Can you work these out from the model? Positions are in its coordinate system, mm. A direction names the side the tool comes from. Coordinates: 2 decimals unless noted, no trailing zeros. Loops run counter-clockwise (first coordinate to the right, second up) from the corner with the lowest first, then second, coordinate; pieces in that order, holes last.
```python
from build123d import *

# Parameters (mm, degrees)
SKETCH_1_R      = 23.5
EXTRUDE_1_DEPTH = 8
EXTRUDE_2_DEPTH = 70
FILLET_1_R      = 3
FILLET_2_R      = 3
EXTRUDE_3_DEPTH = 4


with BuildPart() as part:
    # 草图1 → 凸台-拉伸1 (new body)
    with BuildSketch(Plane.XY):
        with BuildLine():
            Line((30, -32.5), (-30, -32.5))
            Line((-30, -32.5), (-30, 0))
            ThreePointArc((-30, 0), (0, 30), (30, 0))
            Line((30, 0), (30, -32.5))
        make_face()
        Circle(SKETCH_1_R, mode=Mode.SUBTRACT)
    extrude(amount=EXTRUDE_1_DEPTH)

    # 草图2 → 凸台-拉伸2 (add)
    with BuildSketch(Plane(origin=(30, 0, 0), x_dir=(0, 0, -1), z_dir=(1, 0, 0))):
        Polygon((1, -32.5), (4, -32.5), (4, -27.5), (-12, -27.5), (-12, -32.5), (-9, -32.5), (-9, -42.5), (-19, -42.5), (-19, -47.5), (11, -47.5), (11, -42.5), (1, -42.5), align=None)
    extrude_2 = extrude(amount=-EXTRUDE_2_DEPTH)

    # 镜向1: 凸台-拉伸2 across plane
    add(extrude_2.mirror(Plane.ZY))

    # 圆角1
    fillet_1_edges = [part.edges().sort_by_distance(p)[0] for p in [
        (30, -13.75, 0),
        (30, -13.75, 8),
        (0, -27.5, 0),
        (-30, -27.5, 4),
        (0, -27.5, 8),
        (0, 30, 8),
        (-30, -13.75, 0),
        (0, 30, 0),
        (30, -27.5, 4),
        (-30, -13.75, 8),
    ]]
    fillet(fillet_1_edges, radius=FILLET_1_R)

    # 圆角2
    fillet_2_edges = [part.edges().sort_by_distance(p)[0] for p in [
        (-40, -47.5, 4),
        (0, -47.5, -11),
        (0, -47.5, 19),
        (40, -47.5, 4),
    ]]
    fillet(fillet_2_edges, radius=FILLET_2_R)

    # 草图4 → 凸台-拉伸3 (add, symmetric)
    with BuildSketch(Plane.XY.offset(4)):
        with BuildLine():
            Line((7.5, -47.5), (5, -47.5))
            Line((5, -47.5), (5, -52.5))
            ThreePointArc((5, -52.5), (0, -57.5), (-5, -52.5))
            Line((-5, -52.5), (-5, -47.5))
            Line((-5, -47.5), (-7.5, -47.5))
            Line((-7.5, -47.5), (-7.5, -52.5))
            ThreePointArc((-7.5, -52.5), (-6.18240924, -56.745917567), (-2.692582404, -59.5))
            Line((-2.692582404, -59.5), (2.692582404, -59.5))
            ThreePointArc((2.692582404, -59.5), (6.18240924, -56.745917567), (7.5, -52.5))
            Line((7.5, -52.5), (7.5, -47.5))
        make_face()
    extrude(amount=EXTRUDE_3_DEPTH, both=True)


solid = part.part
```
(1) I want a section at C-C on x = -35. Write out the boundary of the cut face in (y, z), then the cut area to 3 significant figures.
Check values:
outline: (-47.5, -8) arc R3 ccw to (-44.5, -11) - (-42.5, -11) - (-42.5, -1) - (-32.5, -1) - (-32.5, -4) - (-27.5, -4) - (-27.5, 12) - (-32.5, 12) - (-32.5, 9) - (-42.5, 9) - (-42.5, 19) - (-44.5, 19) arc R3 ccw to (-47.5, 16) - close
area: 326 mm2
(2) If we mould it in two halves opening along Y, with no side actions, what happens to faces 5 (the flat face through (-1.8, -57.4, 0)), 6 (the cylindrical face through (0.38, -26.64, -0.9)), 7 (the flat face through (-1, -42.5, 14))? For each: released by +Y, released by -Y, zero draft, split by the parting line, or undercut.
Check values:
face 5: zero draft
face 6: released by +Y
face 7: undercut
(3) I want a section at B-B on y = -3.5. Write out the boundary of the cut face in (x, z), then the cut area to 3 significant figures.
Check values:
outline: (-30, 3) arc R3 ccw to (-27, 0) - (-23.24, 0) - (-23.24, 8) - (-27, 8) arc R3 ccw to (-30, 5) - close; (23.24, 0) - (27, 0) arc R3 ccw to (30, 3) - (30, 5) arc R3 ccw to (27, 8) - (23.24, 8) - close
area: 100 mm2
(4) If I drill on probe 1 along Y at (x, z) = (0, 5); probe 2 along X at (y, z) = (-51, 0.5); probe 3 along Y at (x, z) = (-16.5, 9.5), over which ranges is the centre line in solid material (lowest first)?
Check values:
probe 1: y = -59.5 to -57.5, -47.5 to -23.5, 23.5 to 30
probe 2: x = -7.5 to -5, 5 to 7.5
probe 3: y = -47.5 to -42.5, -32.5 to -27.1
(5) Which directions (+Z, -Z, +X, -X, +Y, -Y) give clear straight access to the entire face, cutting with the end or side of a thin tool? Please do faces 1 (the cylindrical face through (29.1, -12.42, 0.86)), 2 (the cylindrical face through (-29.1, -12.08, 7.14)), 3 (the flat face through (5, -50, 4)), 4 (the flat face through (-7.5, -50, 4)).
Check values:
face 1: -Z, +X, +Y
face 2: +Z, -X, +Y
face 3: +Z, -Z
face 4: +Z, -Z, -X, -Y
(6) I want a section at A-A on x = 0. State how many separate pieces and enclosed holes the cut face has, then the cut area to 3 significant figures.
Check values:
separate pieces: 3
enclosed holes: 0
area: 426 mm2
(7) I'm going to push flat-ended pins straight in: pin 1 (12 mm diameter, centred on x = -6, z = 15, fed in from -Y); pin 2 (8 mm diameter, centred on x = 3, z = 6, fed in from +Y); pin 3 (5.5 mm diameter, centred on y = -51, z = 4.5, fed in from -X); pin 4 (12 mm diameter, centred on x = 9.5, y = -45.5, fed in from +Z). Where does each tip first touch, or does it pass through?
Check values:
pin 1: stops at y = -47.5
pin 2: stops at y = 30
pin 3: stops at x = -7.5
pin 4: stops at z = 19
(8) I want a section at D-D on z = -6. Write out the boundary of the cut face in (x, y), then the cut area to 3 significant figures.
Check values:
outline: (-40, -44.5) arc R3 ccw to (-37, -47.5) - (37, -47.5) arc R3 ccw to (40, -44.5) - (40, -42.5) - (-40, -42.5) - close
area: 396 mm2
